```python
from build123d import *

# Parameters (mm, degrees)
SKETCH_W        = 65
SKETCH_H        = 20
PAD_DEPTH       = 5
SKETCH001_W     = 5
SKETCH001_H     = 20
SKETCH001_W_2   = 31.7
PAD001_DEPTH    = 5
POCKET_DEPTH    = 31.7
SKETCH003_R     = 5
PAD002_DEPTH    = 15
SKETCH004_R     = 3.3
POCKET001_DEPTH = 15


with BuildPart() as part:
    # Sketch → Pad (new body)
    with BuildSketch(Plane.XY):
        with Locations((2.5, 0)):
            Rectangle(SKETCH_W, SKETCH_H)
    extrude(amount=PAD_DEPTH)

    # Sketch001 → Pad001 (new body)
    with BuildSketch(Plane.XY.offset(5)):
        with Locations((-27.5, 0)):
            Rectangle(SKETCH001_W, SKETCH001_H)
        with Locations((19.15, 0)):
            Rectangle(SKETCH001_W_2, SKETCH001_H)
    extrude(amount=PAD001_DEPTH)

    # Sketch002 → Pocket (cut)
    with BuildSketch(Plane.YZ.offset(35)):
        with BuildLine():
            Line((-2.73443, 10), (-2.73443, 6.487833))
            ThreePointArc((-2.73443, 6.487833), (0, 3.753403), (2.73443, 6.487833))
            Line((2.73443, 10), (2.73443, 6.487833))
            Line((-2.73443, 10), (2.73443, 10))
        make_face()
    extrude(amount=-POCKET_DEPTH, mode=Mode.SUBTRACT)

    # Sketch003 → Pad002 (new body)
    with BuildSketch(Plane.XZ.offset(10)):
        with Locations((30, 5)):
            Circle(SKETCH003_R)
    extrude(amount=PAD002_DEPTH)

    # Sketch004 → Pocket001 (cut)
    with BuildSketch(Plane.XZ.offset(25)):
        with Locations((30, 5)):
            Circle(SKETCH004_R)
    extrude(amount=-POCKET001_DEPTH, mode=Mode.SUBTRACT)


solid = part.part
```
Build history of the part. All positions in model axes, mm. A direction names the side the tool comes from. Give positions to 0.01 mm unless a question says otherwise; leave off trailing zeros. Loops run counter-clockwise (first coordinate to the right, second up) from the corner with the lowest first, then second, coordinate; pieces in that order, holes last.
1) Band-saw the part on D-D on y = -19.5. List the corners of the cut face in (x, z), then the cut area to 3 significant figures.
Values follow:
outline: circle Ø10 at (30, 5); hole circle Ø6.6 at (30, 5)
area: 44.3 mm2
2) 3-axis set-ups, long thin cutter, end or side, ignore diameter. For faces 1 (the face through (34, -10, 9)), 2 (the face through (30, -10, 5)), 3 (the face through (-25, 0, 7)), 4 (the face through (19, -2.734, 8)), 5 (the face through (34, -10, 1)): which of +Z, -Z, +X, -X, +Y, -Y reach the whole face in a straight line?
Values follow:
face 1: +Z, +X, -Y
face 2: -Y
face 3: +Z, +Y, -Y
face 4: +Z, +X
face 5: -Z, +X, -Y
3) Two-plate mould, pull along X, no slides. Class faces 6 (the face through (25, -17, 5)), 7 (the face through (35, 0, 3)), 8 (the face through (-11, 0, 5)): released by +X, released by -X, zero draft, split by the parting line, or undercut.
Values follow:
face 6: split by the parting line
face 7: released by +X
face 8: undercut
4) Probe line 1 along Z through (x, y) = (30, -19); line 2 along X through (y, z) = (-3.5, 7.5); line 3 along Z through (x, y) = (2, 5). List the from-to ranges inside material, lowest first.
Values follow:
line 1: z = 0 to 1.7, 8.3 to 10
line 2: x = -30 to -25, 3.3 to 35
line 3: z = 0 to 5
5) Band-saw the part on B-B on y = 0. List the corners of the cut face in (x, z).
Values follow:
outline: (-30, 0) - (35, 0) - (35, 3.75) - (3.3, 3.75) - (3.3, 5) - (-25, 5) - (-25, 10) - (-30, 10) - close
6) Band-saw the part on A-A on z = 7.25. List the corners of the cut face in (x, y).
Values follow:
outline: (-30, -10) - (-25, -10) - (-25, 10) - (-30, 10) - close; (3.3, -10) - (25.53, -10) - (25.53, -25) - (27.59, -25) - (27.59, -10) - (32.41, -10) - (32.41, -25) - (34.47, -25) - (34.47, -10) - (35, -10) - (35, -2.73) - (3.3, -2.73) - close; (3.3, 2.73) - (35, 2.73) - (35, 10) - (3.3, 10) - close
7) Drop flat-ended pins along their axis: P1, Ø6, axis at x = 30, z = 5, coming from the -Y side; P2, Ø1.4, axis at y = 0, z = 4, coming from the +X side. Give the stop position or say it passes through.
Values follow:
P1: stops at y = -10
P2: stops at x = 35
8) Band-saw the part on C-C on x = 28. List the corners of the cut face in (y, z).
Values follow:
outline: (-25, 0.42) - (-10, 0.42) - (-10, 0) - (10, 0) - (10, 10) - (2.73, 10) - (2.73, 6.49) arc R2.73 cw to (-2.73, 6.49) - (-2.73, 10) - (-10, 10) - (-10, 9.58) - (-25, 9.58) - (-25, 7.62) - (-10, 7.62) - (-10, 2.38) - (-25, 2.38) - close
